Autodesk Inventor part; units mm, degrees
ref_plane "YZ Plane" through (0, 0, 0) normal (1, 0, 0) x (0, 1, 0)
ref_plane "XZ Plane" through (0, 0, 0) normal (0, 1, 0) x (-1, 0, 0)
ref_plane "XY Plane" through (0, 0, 0) normal (0, 0, 1) x (1, 0, 0)
sketch "Sketch1" plane through (0, 0, 0) normal (0, 1, 0) x (-1, 0, 0)
  circle A0 centre (0, 0) radius 3.15
  circle A1 centre (0, 0) radius 6
  dimension "d0" = 6.3
  dimension "d2" = 12
extrude "Extrusion1" add sketch "Sketch1" along normal blind 11
sketch "Sketch2" plane through (0, 11, 0) normal (0, 1, 0) x (1, 0, 0)
  circle A0 centre (0, 0) radius 2.6288
  circle A1 centre (0, 0) radius 3.15
  circle A2 centre (0, 0) radius 8.5
  dimension "d5" = 17
extrude "Extrusion2" add sketch "Sketch2" against normal blind 3 contours A2
ref_plane "Work Plane1" through (0, 4, 0) normal (0, -1, 0) x (1, 0, 0)
mirror "Mirror1" about plane through (0, 4, 0) normal (0, -1, 0) of "Extrusion2"
ref_plane "Work Plane2" through (0, 4, 0) normal (0, -1, 0) x (1, 0, 0)
properties part number "Belt tensor V2"
The listing builds one solid part. Answer for the finished solid, in the listing's coordinates (mm). A direction names the side the tool comes from. Give positions to 0.01 mm unless a question says otherwise; leave off trailing zeros. Order: outer loops, then holes, each group sorted by start corner. A loop starts at its lowest first (then second) coordinate and runs counter-clockwise, first axis right, second up.
1) For faces 1 (the face through (-2, 0, -6)), 2 (the face through (4.57, 9.521, -7.167)), determine the directions among +Z, -Z, +X, -X, +Y, -Y from which every point of the face is accessible in a straight line to the end or side of a thin tool.
Reported:
face 1: none
face 2: +Y, -Y
2) Determine the mould class of faces 3 (the face through (2, 8, -6)), 4 (the face through (4, 11, 0)), 5 (the face through (-4, -3, 0)) for opening direction Y: pulls with the +Y half, pulls with the -Y half, needs draft (parallel to the pull), parting line crosses it, or undercut.
Reported:
face 3: undercut
face 4: pulls with the +Y half
face 5: pulls with the -Y half
3) Find section A-A on z = 1. Write down the section's boundary in (x, y), then the cut area to 3 significant figures.
Reported:
outline: (-8.44, -3) - (-2.99, -3) - (-2.99, 11) - (-8.44, 11) - (-8.44, 8) - (-5.92, 8) - (-5.92, 0) - (-8.44, 0) - close; (2.99, -3) - (8.44, -3) - (8.44, 0) - (5.92, 0) - (5.92, 8) - (8.44, 8) - (8.44, 11) - (2.99, 11) - close
area: 112 mm2
4) Find section B-B on x = 7. Write down the section's boundary in (y, z), then the cut area to 3 significant figures.
Reported:
outline: (-3, -4.82) - (0, -4.82) - (0, 4.82) - (-3, 4.82) - close; (8, -4.82) - (11, -4.82) - (11, 4.82) - (8, 4.82) - close
area: 57.9 mm2
5) Find section D-D on y = 1.5. Write down the section's boundary in (x, z), then the cut area to 3 significant figures.
Reported:
outline: circle Ø12 at (0, 0); hole circle Ø6.3 at (0, 0)
area: 81.9 mm2
6) Consider line 1 along Y through (x, z) = (5.5, -5); line 2 along Z through (x, y) = (0, 6.5). Determine where each line is inside the solid, lowest interval first.
Reported:
line 1: y = -3 to 0, 8 to 11
line 2: z = -6 to -3.15, 3.15 to 6
7) Given P1, Ø6, axis at y = 1.5, z = -4, coming from the +X side; P2, Ø3, axis at y = 5, z = -2, coming from the +X side; P3, Ø1.5, axis at y = 2, z = -5, coming from the +X side, each flat-ended and moving along its own axis, determine where each tip first touches the part or whether it passes through.
Reported:
P1: stops at x = 8.38
P2: stops at x = 5.98
P3: stops at x = 4.24
